Geometry: see drawing. Coordinates: mm, zero at the bounding-box minimum. A direction names the side the tool comes from. Coordinates: 2 decimals unless noted, no trailing zeros. Write each loop counter-clockwise with the first axis right and the second up, starting at its lowest first coordinate (ties: lowest second). Pieces come first, ordered by that corner, then holes. Notation, with made-up numbers: (32.5, 59) - (52.5, 59) arc R10 cw to (52.5, 75) - close; hole circle Ø10 at (19, 66.25). An arc over 180 degrees is marked (long way). Use a Markdown table: item, result. Add a question column.
Q1. Section query A-A (y = 15.5). Return the cut outline in (x, z), then the cut area to 3 significant figures.
Q2. Section query D-D (z = 124.5). Return the cut outline in (x, y), then the cut area to 3 significant figures.
Q3. Pin query (flat end, axial travel): P1, Ø3, axis at x = 6.35, z = 6.35, coming from the -Y side; P2, Ø4, axis at x = 202.5, z = 21, coming from the -Y side. Return the tip coordinate at first contact, or that it passes through.
Q4. Set-up query: the marked faces 1 and 2. Return all of +Z, -Z, +X, -X, +Y, -Y with unobstructed straight access to the full face (end or side cutting, diameter ignored); none if empty.
Q5. Material intervals for probe 1 along Z at (x, y) = (247.65, 7.25); probe 2 along X at (y, z) = (18.5, 146.05); probe 3 along X at (y, z) = (12.5, 18), sorted ascending. Write a range as from..to.
Q6. Mould query, pull axis X, two halves, no side actions, for the marked faces 3, 4 and 5. Classes: released by +X, released by -X, zero draft, split by the parting line, or undercut.
Q7. Section query B-B (x = 247.65). Return the cut outline in (y, z).
Q8. Section query C-C (x = 181.5). Return the cut outline in (y, z).
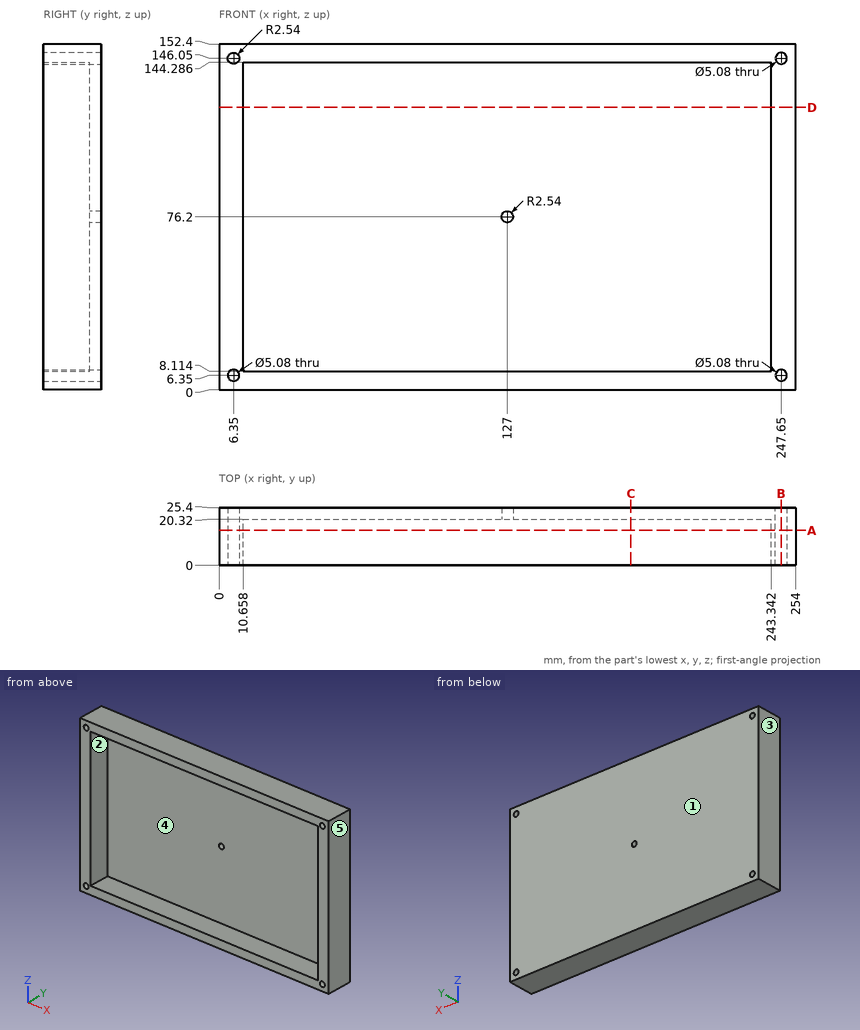
Values follow:
| question | item | result |
|---|---|---|
| 1 | outline | (0, 0) - (254, 0) - (254, 152.4) - (0, 152.4) - close; hole circle Ø5.08 at (6.35, 6.35); hole circle Ø5.08 at (6.35, 146.05); hole (10.66, 8.11) - (243.34, 8.11) - (243.34, 144.29) - (10.66, 144.29) - close; hole circle Ø5.08 at (247.65, 6.35); hole circle Ø5.08 at (247.65, 146.05) |
| 1 | area | 6,940 mm2 |
| 2 | outline | (0, 0) - (10.66, 0) - (10.66, 20.32) - (243.34, 20.32) - (243.34, 0) - (254, 0) - (254, 25.4) - (0, 25.4) - close |
| 2 | area | 1,720 mm2 |
| 3 | P1 | through |
| 3 | P2 | y = 20.32 |
| 4 | face 1 | +Z, -Z, +X, -X, +Y |
| 4 | face 2 | -Y |
| 5 | probe 1 | 0..3.81, 8.89..143.51, 148.59..152.4 |
| 5 | probe 2 | 0..3.81, 8.89..245.11, 250.19..254 |
| 5 | probe 3 | 0..10.66, 243.34..254 |
| 6 | face 3 | released by -X |
| 6 | face 4 | undercut |
| 6 | face 5 | released by +X |
| 7 | outline | (0, 0) - (25.4, 0) - (25.4, 3.81) - (0, 3.81) - close; (0, 8.89) - (25.4, 8.89) - (25.4, 143.51) - (0, 143.51) - close; (0, 148.59) - (25.4, 148.59) - (25.4, 152.4) - (0, 152.4) - close |
| 8 | outline | (0, 0) - (25.4, 0) - (25.4, 152.4) - (0, 152.4) - (0, 144.29) - (20.32, 144.29) - (20.32, 8.11) - (0, 8.11) - close |
